Could you check a few things on this model? Use its own coordinates, in mm. A direction names the side the tool comes from. Give positions to 0.01 mm unless a question says otherwise; leave off trailing zeros. Loops run counter-clockwise (first coordinate to the right, second up) from the corner with the lowest first, then second, coordinate; pieces in that order, holes last. Notation, with made-up numbers: (44, -37) -> (102, -37) arc R11 ccw to (102, -32) -> close; hole circle Ø7 at (19, -13). An arc over 180 degrees is marked (long way). Write item = value, one per line. Start each with the question number.
1) I want a section at A-A (x = -25). List the corners of the cut face in (y, z) for me, and give its area (3 significant figures).
2) I need wall thicknesses on probe 1 along Y at (x, z) = (-25, -2); probe 2 along Z at (x, y) = (-18, -44.5). Which ranges of each line are inside material? Lowest first, please. Write a range as from..to.
3) On a 3-axis mill with a long thin cutter (end or side, diameter ignored), from which of +Z, -Z, +X, -X, +Y, -Y can I reach the whole of each face in a straight line? I mean faces 4 (the face through (0, -25, -25)), 5 (the face through (-30, -25, -46)). Say none if no direction works.
4) If we mould it in two halves opening along Z, with no side actions, what happens to faces 1 (the face through (-3, -50, -25)), 2 (the face through (-25, -19, -50)), 3 (the face through (-46, -25, -25))? For each: +Z half, -Z half, draft (parallel to the pull), parting line (faces both ways), or undercut.
5) I want a section at C-C (z = -6.5). List the corners of the cut face in (x, y) for me.
6) I want a section at D-D (y = -33). List the corners of the cut face in (x, z) for me.
7) I want a section at B-B (x = -13). List the corners of the cut face in (y, z) for me, and give its area (3 significant figures).
from build123d import *

# Parameters (mm, degrees)
F0_W     = 50
F0_H     = 50
F0_W_2   = 42
F0_H_2   = 42
F1_DEPTH = 50
F2_R     = 6
F3_DEPTH = 50.001


with BuildPart() as f1:
    # F0 (on Front) → F1 (new body)
    with BuildSketch(Plane.XZ):
        with Locations((-25, -25)):
            Rectangle(F0_W, F0_H)
        with Locations((-25, -25)):
            Rectangle(F0_W_2, F0_H_2, mode=Mode.SUBTRACT)
    extrude(amount=F1_DEPTH)

    # F2 (on face) → F3 (cut, through all)
    with BuildSketch(Plane.XY):
        with Locations((-25, -30)):
            Circle(F2_R)
    extrude(amount=-F3_DEPTH, mode=Mode.SUBTRACT)


solid = f1.part
Answer list:
q1.outline = (-50, -50) -> (-36, -50) -> (-36, -46) -> (-50, -46) -> close; (-50, -4) -> (-36, -4) -> (-36, 0) -> (-50, 0) -> close; (-24, -50) -> (0, -50) -> (0, -46) -> (-24, -46) -> close; (-24, -4) -> (0, -4) -> (0, 0) -> (-24, 0) -> close
q1.area = 304 mm^2
q2.probe_1 = -50..-36, -24..0
q2.probe_2 = -50..-46, -4..0
q3.face_4 = +Z, -Z, +X, +Y, -Y
q3.face_5 = +Y, -Y
q4.face_1 = draft
q4.face_2 = -Z half
q4.face_3 = undercut
q5.outline = (-50, -50) -> (-46, -50) -> (-46, 0) -> (-50, 0) -> close; (-4, -50) -> (0, -50) -> (0, 0) -> (-4, 0) -> close
q6.outline = (-50, -50) -> (-30.2, -50) -> (-30.2, -46) -> (-46, -46) -> (-46, -4) -> (-30.2, -4) -> (-30.2, 0) -> (-50, 0) -> close; (-19.8, -50) -> (0, -50) -> (0, 0) -> (-19.8, 0) -> (-19.8, -4) -> (-4, -4) -> (-4, -46) -> (-19.8, -46) -> close
q7.outline = (-50, -50) -> (0, -50) -> (0, -46) -> (-50, -46) -> close; (-50, -4) -> (0, -4) -> (0, 0) -> (-50, 0) -> close
q7.area = 400 mm^2
